from build123d import *

# Parameters (mm, degrees)
FILLET1_R       = 0.2
HEX_START       = -1.9
HEX_2_DEPTH     = 1.9
THDSCHPAT_COUNT = 20
THDSCHPAT_PITCH = 0.765


with BuildPart() as part:
    # BodySke → BaseBody (revolve)
    with BuildSketch(Plane.XY, mode=Mode.PRIVATE) as basebody_sk:
        Polygon((0, 0), (0, 4.875), (0.725, 4.875), (3.1, 2.5), (19.555, 2.5), (20, 2.055), (20, 0), align=None)
    revolve(basebody_sk.sketch.rotate(Axis((0, 0, 0), (1, 0, 0)), 90), axis=Axis((0, 0, 0), (1, 0, 0)))

    # Fillet1
    fillet1_edges = [part.edges().sort_by_distance(p)[0] for p in [
        (3.1, 0, -2.5),
    ]]
    fillet(fillet1_edges, radius=FILLET1_R)

    # Hex 2: read off the stored shape, not the designer's step
    # Hex 2 outline → Hex 2 (cut)
    with BuildSketch(Plane.ZY.offset(HEX_START)):
        Polygon((-1.5, -0.866025404), (0, -1.732050808), (1.5, -0.866025404), (1.5, 0.866025404), (0, 1.732050808), (-1.5, 0.866025404), align=None)
    extrude(amount=HEX_2_DEPTH, mode=Mode.SUBTRACT)

    # Hex 2 2 outline → Hex 2 2 (revolve, cut)
    with BuildSketch(Plane.YX):
        Polygon((1.5, 1.9), (0, 2.766025404), (0, 1.9), align=None)
    revolve(axis=Axis((0, 0, 0), (1, 0, 0)), mode=Mode.SUBTRACT)

    # ThdSchSke → ThreadSchematic (revolve, cut)
    with BuildSketch(Plane.XY, mode=Mode.PRIVATE) as threadschematic_sk:
        Polygon((4.700001, -2.055), (4.388408645, -2.5), (4.388408645, -3.125), (5.011593355, -3.125), (5.011593355, -2.5), align=None)
    threadschematic = revolve(threadschematic_sk.sketch.rotate(Axis((-3.175, 0, 0), (1, 0, 0)), 270), axis=Axis((-3.175, 0, 0), (1, 0, 0)), mode=Mode.SUBTRACT)

    # ThdSchPat: ThreadSchematic ×20
    with Locations(*[(i * THDSCHPAT_PITCH, 0, 0) for i in range(1, THDSCHPAT_COUNT)]):
        add(threadschematic, mode=Mode.SUBTRACT)


solid = part.part
Source: CAD feature listing. Evaluate the final solid. Frame: model axes, mm. A direction names the side the tool comes from. Give positions to 0.01 mm unless a question says otherwise; leave off trailing zeros. Return JSON: item names as keys, results as strings. Group by question number.
1) Material intervals for line 1 along Z through (x, y) = (1.5, 1); line 2 along X through (y, z) = (-4, 1.75); line 3 along X through (y, z) = (-1.25, -0.75), sorted ascending. Write a range as [from, to].
2) Pull-direction query (Z, two-part tool) for faces 3 (the face through (20, 0, 0)), 4 (the face through (0.963, -1.305, 0.74)), 5 (the face through (0.368, -4.834, -0.635)); classes: pulls with the +Z half, pulls with the -Z half, needs draft (parallel to the pull), parting line crosses it, or undercut.
3) Set-up query: faces 1 (the face through (0, 0, -2)), 2 (the face through (1, 0, 1.5)). Return all of +Z, -Z, +X, -X, +Y, -Y with unobstructed straight access to the full face (end or side cutting, diameter ignored); none if empty.
4) Pin query (flat end, axial travel): P1, Ø0.9, axis at x = 1.5, y = 0, coming from the -Z side; P2, Ø1.4, axis at x = 1.5, y = 0, coming from the +Z side; P3, Ø4, axis at x = 10, z = -3.5, coming from the -Y side; P4, Ø1.5, axis at x = 8, y = -3.5, coming from the -Z side. Return the tip coordinate at first contact, or that it passes through.
Recorded:
{
 "1": {"line 1": "z = [-3.98, -1.27], [1.27, 3.98]", "line 2": "x = [0, 1.23]", "line 3": "x = [1.92, 20]"},
 "2": {"face 3": "needs draft", "face 4": "undercut", "face 5": "parting line crosses it"},
 "3": {"face 1": "+Z, -Z, -X, +Y, -Y", "face 2": "-X"},
 "4": {"P1": "stops at z = -4.55", "P2": "stops at z = 4.8", "P3": "stops at y = -1.99", "P4": "passes through"}
}
